Verification items for the finished model (mm, model axes). A direction names the side the tool comes from. Round coordinates to 2 decimals unless told otherwise and drop trailing zeros. Order: outer loops, then holes, each group sorted by start corner. A loop starts at its lowest first (then second) coordinate and runs counter-clockwise, first axis right, second up. Notation, with made-up numbers: M 2.5,-14 L 57.5,-14 A23 cw 57.5,23 Z; hole C 39,21.25 d2. An arc over 180 degrees is marked long. Answer as a JSON object with one key per item and string values. Group by question number.
```python
from build123d import *

# Parameters (mm, degrees)
SKETCH1_W           = 3.4
SKETCH1_H           = 6.1
SKETCH1_W_2         = 12
SKETCH1_H_2         = 22.665
SKETCH1_R           = 1.475
BOSS_EXTRUDE1_DEPTH = 5.58


with BuildPart() as part:
    # Sketch1 → Boss-Extrude1 (new body)
    with BuildSketch(Plane.XY):
        with BuildLine():
            Line((708.295729089, 432.614671907), (715.695729089, 432.614671907))
            Line((715.695729089, 432.614671907), (723.095729089, 432.614671907))
            ThreePointArc((723.095729089, 432.614671907), (726.631262995, 434.079138001), (728.095729089, 437.614671907))
            Line((728.095729089, 437.614671907), (728.095729089, 498.294671907))
            ThreePointArc((728.095729089, 498.294671907), (726.631262995, 501.830205812), (723.095729089, 503.294671907))
            Line((723.095729089, 503.294671907), (715.695729089, 503.294671907))
            Line((715.695729089, 503.294671907), (708.295729089, 503.294671907))
            ThreePointArc((708.295729089, 503.294671907), (704.760195183, 501.830205812), (703.295729089, 498.294671907))
            Line((703.295729089, 498.294671907), (703.295729089, 437.614671907))
            ThreePointArc((703.295729089, 437.614671907), (704.760195183, 434.079138001), (708.295729089, 432.614671907))
        make_face()
        with Locations((707.995729089, 463.429671907)):
            Rectangle(SKETCH1_W, SKETCH1_H, mode=Mode.SUBTRACT)
        with Locations((715.695729089, 448.947171907)):
            Rectangle(SKETCH1_W_2, SKETCH1_H_2, mode=Mode.SUBTRACT)
        with Locations((723.395729089, 463.429671907)):
            Rectangle(SKETCH1_W, SKETCH1_H, mode=Mode.SUBTRACT)
        with Locations((707.995729089, 472.479671907)):
            Rectangle(SKETCH1_W, SKETCH1_H, mode=Mode.SUBTRACT)
        with Locations((715.695729089, 467.954671907)):
            Circle(SKETCH1_R, mode=Mode.SUBTRACT)
        with Locations((723.395729089, 472.479671907)):
            Rectangle(SKETCH1_W, SKETCH1_H, mode=Mode.SUBTRACT)
        with Locations((715.695729089, 486.962171907)):
            Rectangle(SKETCH1_W_2, SKETCH1_H_2, mode=Mode.SUBTRACT)
    extrude(amount=BOSS_EXTRUDE1_DEPTH)


solid = part.part
```
Q1. Cross-section at C-C, the plane y = 471. Record the cut outline in (x, z), then the cut area to 3 significant figures.
Q2. Gauge pin test, flat end, axial feed: pin 1 Ø3.5 at (x, y) = (715.7, 467.95) entering from +Z. Record the tip position at first contact, or that the pin passes through.
Q3. Release check for a two-part mould opening along X. For faces 1 (the face through (706.296, 472, 3)), 2 (the face through (716, 498.295, 3)), 3 (the face through (728.096, 468, 3)), 4 (the face through (704.72, 434.12, 2.75)) record: released by +X, released by -X, zero draft, split by the parting line, or undercut.
Q4. Cross-section at A-A, the plane y = 445.5. Record the cut outline in (x, z).
Q5. Cross-section at B-B, the plane x = 712.5. Record the cut outline in (y, z).
Q6. Cross-section at D-D, the plane z = 1.35. Give the number of separate pieces and of enclosed holes in the cut face, then the cut area to 3 significant figures.
Q7. Tool access check on faces 5 (the face through (709.696, 463, 3)), 6 (the face through (704.8, 501.87, 2.75)). Record the directions out of +Z, -Z, +X, -X, +Y, -Y that give a thin tool (end or side, any length) a straight path to the whole face; none if there is none.
Q8. Thickness scan on line 1 (Y direction, x = 712.5, z = 0.95); line 2 (Y direction, x = 715.75, z = 2.1); line 3 (Y direction, x = 708.25, z = 4.1). Record the ranges inside material, lowest first. Write a range as from..to.
Conclusion:
{
 "1": {"outline": "M 703.3,0 L 706.3,0 L 706.3,5.58 L 703.3,5.58 Z; M 709.7,0 L 721.7,0 L 721.7,5.58 L 709.7,5.58 Z; M 725.1,0 L 728.1,0 L 728.1,5.58 L 725.1,5.58 Z", "area": "100 mm2"},
 "2": {"pin 1": "z = 5.58"},
 "3": {"face 1": "undercut", "face 2": "undercut", "face 3": "released by +X", "face 4": "released by -X"},
 "4": {"outline": "M 703.3,0 L 709.7,0 L 709.7,5.58 L 703.3,5.58 Z; M 721.7,0 L 728.1,0 L 728.1,5.58 L 721.7,5.58 Z"},
 "5": {"outline": "M 432.61,0 L 437.61,0 L 437.61,5.58 L 432.61,5.58 Z; M 460.28,0 L 475.63,0 L 475.63,5.58 L 460.28,5.58 Z; M 498.29,0 L 503.29,0 L 503.29,5.58 L 498.29,5.58 Z"},
 "6": {"separate pieces": "1", "enclosed holes": "7", "area": "1,100 mm2"},
 "7": {"face 5": "+Z, -Z", "face 6": "+Z, -Z, -X, +Y"},
 "8": {"line 1": "432.61..437.61, 460.28..475.63, 498.29..503.29", "line 2": "432.61..437.61, 460.28..466.48, 469.43..475.63, 498.29..503.29", "line 3": "432.61..460.38, 466.48..469.43, 475.53..503.29"}
}
